Geometry: final body of the model. Coordinates: model frame, mm. A direction names the side the tool comes from. Give positions to 0.01 mm unless a question says otherwise; leave off trailing zeros. Order: outer loops, then holes, each group sorted by start corner. A loop starts at its lowest first (then second) coordinate and runs counter-clockwise, first axis right, second up. Notation, with made-up numbers: (6.5, 31) -> (39.5, 31) arc R11 cw to (39.5, 47) -> close; hole circle Ø11 at (38.25, 8). An arc over 180 degrees is marked (long way). One line per question, with ' | ' between items.
Autodesk Inventor part; units mm, degrees
ref_plane "YZ Plane" through (0, 0, 0) normal (1, 0, 0) x (0, 1, 0)
ref_plane "XZ Plane" through (0, 0, 0) normal (0, 1, 0) x (-1, 0, 0)
ref_plane "XY Plane" through (0, 0, 0) normal (0, 0, 1) x (1, 0, 0)
sketch "スケッチ1" plane through (0, 0, 0) normal (0, 0, 1) x (1, 0, 0)
  line L0 (16.9587, -21.15) -> (-16.9587, -21.15)
  line L1 (-21.15, -16.9587) -> (-21.15, 16.9587)
  line L2 (-16.9587, 21.15) -> (16.9587, 21.15)
  line L3 (21.15, 16.9587) -> (21.15, -16.9587)
  line L4 (21.15, -21.15) -> (-21.15, 21.15) construction
  line L5 (-21.15, -21.15) -> (21.15, 21.15) construction
  line L6 (-16.9587, 21.15) -> (-21.15, 16.9587)
  line L7 (-21.15, -16.9587) -> (-16.9587, -21.15)
  line L8 (16.9587, -21.15) -> (21.15, -16.9587)
  line L9 (21.15, 16.9587) -> (16.9587, 21.15)
  point P0 (0, 0)
  dimension "d4" = 360
  dimension "d0" = 42.3
  dimension "d1" = 42.3
extrude "押し出し1" add sketch "スケッチ1" along normal blind 48
sketch "スケッチ2" plane through (0, 0, 48) normal (0, 0, 1) x (1, 0, 0)
  line L0 (15.5, -15.5) -> (-15.5, -15.5)
  line L1 (-15.5, -15.5) -> (-15.5, 15.5)
  line L2 (-15.5, 15.5) -> (15.5, 15.5)
  line L3 (15.5, 15.5) -> (15.5, -15.5)
  line L4 (15.5, -15.5) -> (-15.5, 15.5) construction
  line L5 (-15.5, -15.5) -> (15.5, 15.5) construction
  point P0 (0, 0)
  point P1 (15.5, 15.5)
  dimension "d8" = 31
  dimension "d9" = 31
hole "穴1" at (-15.5, 15.5, 48) at (15.5, 15.5, 48) at (15.5, -15.5, 48) at (-15.5, -15.5, 48) direction (0, 0, -1) diameter 2.459 depth 4.5
sketch "スケッチ3" plane through (0, 0, 48) normal (0, 0, 1) x (1, 0, 0)
  circle A0 centre (0, 0) radius 11
  dimension "d17" = 22
extrude "押し出し2" add sketch "スケッチ3" along normal blind 2
sketch "スケッチ4" plane through (0, 0, 50) normal (0, 0, 1) x (1, 0, 0)
  circle A0 centre (0, 0) radius 2.5
  dimension "d20" = 5
extrude "押し出し3" add sketch "スケッチ4" along normal blind 22
properties part number "ステッピングモータ"
1) Contact query for flat-ended pins moving along their axis: pin 1 Ø1.2 at (x, y) = (-15, -15) entering from +Z; pin 2 Ø0.7 at (x, y) = (15, 15) entering from +Z; pin 3 Ø6.5 at (x, y) = (2, 5.5) entering from +Z. Output: stop coordinate, or through.
Check result:
pin 1: stops at z = 48 | pin 2: stops at z = 43.5 | pin 3: stops at z = 50
2) Material intervals for probe 1 along X at (y, z) = (-15.5, 46.25); probe 2 along X at (y, z) = (15, 47), sorted ascending. Write a range as from..to.
Check result:
probe 1: x = -21.15..-16.73, -14.27..14.27, 16.73..21.15 | probe 2: x = -21.15..-16.62, -14.38..14.38, 16.62..21.15
3) Section C-C on y = 0. Return loops of the section in (x, z).
Check result:
outline: (-21.15, 0) -> (21.15, 0) -> (21.15, 48) -> (11, 48) -> (11, 50) -> (2.5, 50) -> (2.5, 72) -> (-2.5, 72) -> (-2.5, 50) -> (-11, 50) -> (-11, 48) -> (-21.15, 48) -> close
4) Set-up query: faces 1 (the cylindrical face through (-0.54, 2.44, 60.85)), 2 (the flat face through (0, 0, 72)). Return all of +Z, -Z, +X, -X, +Y, -Y with unobstructed straight access to the full face (end or side cutting, diameter ignored); none if empty.
Check result:
face 1: +Z | face 2: +Z, +X, -X, +Y, -Y
5) Section D-D on x = -4.5. Return loops of the section in (y, z), plus the area to 3 significant figures.
Check result:
outline: (-21.15, 0) -> (21.15, 0) -> (21.15, 48) -> (10.04, 48) -> (10.04, 50) -> (-10.04, 50) -> (-10.04, 48) -> (-21.15, 48) -> close | area: 2,070 mm^2
6) Section A-A on z = 42.5. Return loops of the section in (x, y), plus the area to 3 significant figures.
Check result:
outline: (-21.15, -16.96) -> (-16.96, -21.15) -> (16.96, -21.15) -> (21.15, -16.96) -> (21.15, 16.96) -> (16.96, 21.15) -> (-16.96, 21.15) -> (-21.15, 16.96) -> close | area: 1,750 mm^2
7) Section B-B on x = -15.5. Return loops of the section in (y, z), plus the area to 3 significant figures.
Check result:
outline: (-21.15, 0) -> (21.15, 0) -> (21.15, 48) -> (16.73, 48) -> (16.73, 43.5) -> (14.27, 43.5) -> (14.27, 48) -> (-14.27, 48) -> (-14.27, 43.5) -> (-16.73, 43.5) -> (-16.73, 48) -> (-21.15, 48) -> close | area: 2,010 mm^2
